from build123d import *

# Parameters (mm, degrees)
F0_W     = 12.85
F0_H     = 8.35
F1_DEPTH = 4
F2_R     = 3
F3_DEPTH = 6.8
F4_R     = 2.6
F5_DEPTH = 10.801
F6_R     = 0.5
F7_R     = 0.5
F8_SIZE  = 0.49999


# Not quite as in the source:
# - a fillet or chamfer is up to 0.001 mm smaller than in the source, because OpenCascade refuses the exact size


with BuildPart() as f1:
    # F0 (on Top) → F1 (new body)
    with BuildSketch(Plane.XY):
        Rectangle(F0_W, F0_H)
    extrude(amount=F1_DEPTH)

    # F2 (on face) → F3 (join)
    with BuildSketch(Plane.XY.offset(4)):
        Circle(F2_R)
    extrude(amount=F3_DEPTH)

    # F4 (on face) → F5 (cut, through all)
    with BuildSketch(Plane.XY.offset(10.8)):
        Circle(F4_R)
    extrude(amount=-F5_DEPTH, mode=Mode.SUBTRACT)

    # F6
    f6_edges = [f1.edges().sort_by_distance(p)[0] for p in [
        (-6.425, 4.175, 2),
        (6.425, 4.175, 2),
        (6.425, -4.175, 2),
        (-6.425, -4.175, 2),
    ]]
    fillet(f6_edges, radius=F6_R)

    # F7
    f7_edges = [f1.edges().sort_by_distance(p)[0] for p in [
        (0, -4.175, 4),
        (-6.278553, -4.028553, 4),
        (6.278553, -4.028553, 4),
        (-6.425, 0, 4),
        (6.425, 0, 4),
        (-6.278553, 4.028553, 4),
        (6.278553, 4.028553, 4),
        (0, 4.175, 4),
        (-3, 0, 4),
    ]]
    fillet(f7_edges, radius=F7_R)

    # F8 (size 0.5 in the source; OpenCascade refuses exactly that, so slightly less here)
    f8_edges = [f1.edges().sort_by_distance(p)[0] for p in [
        (0, -4.175, 0),
        (-6.278553, -4.028553, 0),
        (6.278553, -4.028553, 0),
        (-6.425, 0, 0),
        (6.425, 0, 0),
        (-6.278553, 4.028553, 0),
        (6.278553, 4.028553, 0),
        (0, 4.175, 0),
        (-2.6, 0, 0),
    ]]
    chamfer(f8_edges, length=F8_SIZE)


solid = f1.part
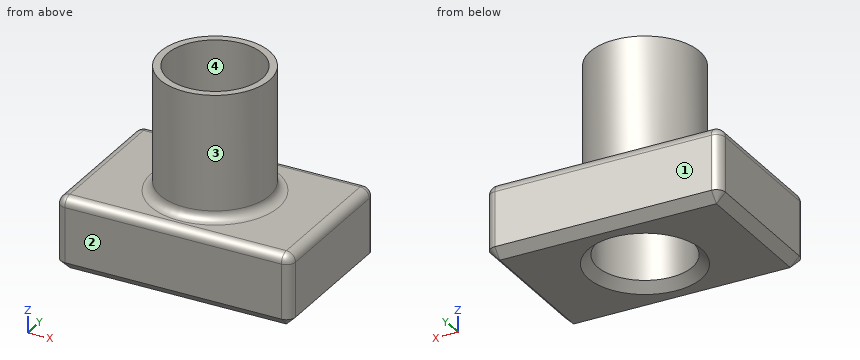
Could you check a few things on this model? Use its own coordinates, in mm. Face numbers are marked on the shaded views. Give positions to 0.01 mm unless a question says otherwise; leave off trailing zeros. Order: outer loops, then holes, each group sorted by start corner. A loop starts at its lowest first (then second) coordinate and runs counter-clockwise, first axis right, second up. Notation, with made-up numbers: M 14,78 L 71,78 A14 ccw 71,102 Z; hole C 61.25,8 d3. An arc over 180 degrees is marked long. One line per question, with ' | ' between items.
1. I want a section at A-A (y = 0). List the corners of the cut face in (x, z) for me (3 decimals).
Results:
outline: M -6.425,0.5 L -5.925,0 L -3.1,0 L -2.6,0.5 L -2.6,10.8 L -3,10.8 L -3,4.5 A0.5 cw -3.5,4 L -5.925,4 A0.5 ccw -6.425,3.5 Z; M 2.6,0.5 L 3.1,0 L 5.925,0 L 6.425,0.5 L 6.425,3.5 A0.5 ccw 5.925,4 L 3.5,4 A0.5 cw 3,4.5 L 3,10.8 L 2.6,10.8 Z
2. We'd pull the mould along Y, two halves only. Please class the marked faces 1, 2, 3 and 4: +Y half, -Y half, draft (parallel to the pull), parting line (faces both ways), or undercut.
Results:
face 1: +Y half | face 2: -Y half | face 3: parting line | face 4: undercut
3. I want a section at C-C (x = 0). List the corners of the cut face in (y, z) for me (3 decimals), and give its area (3 significant figures).
Results:
outline: M -4.175,0.5 L -3.675,0 L -3.1,0 L -2.6,0.5 L -2.6,10.8 L -3,10.8 L -3,4.5 A0.5 cw -3.5,4 L -3.675,4 A0.5 ccw -4.175,3.5 Z; M 2.6,0.5 L 3.1,0 L 3.675,0 L 4.175,0.5 L 4.175,3.5 A0.5 ccw 3.675,4 L 3.5,4 A0.5 cw 3,4.5 L 3,10.8 L 2.6,10.8 Z | area: 17.5 mm²
4. If I drill on line 1 (Y direction, x = 0, z = 3.25) (3 decimals); line 2 (Z direction, x = 3, y = 1.75); line 3 (Y direction, x = 0, z = 5.5), over which ranges is the centre line in solid material (lowest first)?
Results:
line 1: -4.175 to -2.6, 2.6 to 4.175 | line 2: 0 to 4 | line 3: -3 to -2.6, 2.6 to 3
5. I want a section at B-B (z = 2). List the corners of the cut face in (x, y) for me (3 decimals).
Results:
outline: M -6.425,-3.675 A0.5 ccw -5.925,-4.175 L 5.925,-4.175 A0.5 ccw 6.425,-3.675 L 6.425,3.675 A0.5 ccw 5.925,4.175 L -5.925,4.175 A0.5 ccw -6.425,3.675 Z; hole C 0,0 d5.2
6. I want a section at D-D (x = 5). List the corners of the cut face in (y, z) for me (3 decimals).
Results:
outline: M -4.175,0.5 L -3.675,0 L 3.675,0 L 4.175,0.5 L 4.175,3.5 A0.5 ccw 3.675,4 L -3.675,4 A0.5 ccw -4.175,3.5 Z
7. I'm going to push a flat-ended pin straight in: pin 1 (4 mm diameter, centred on x = 0, y = 0, fed in from +Z) (3 decimals). Where does the tip first touch, or does it pass through?
Results:
pin 1: through
